Can you work these out from the model? Positions are in its coordinate system, mm. A direction names the side the tool comes from. Give positions to 0.01 mm unless a question says otherwise; leave off trailing zeros. Loops run counter-clockwise (first coordinate to the right, second up) from the corner with the lowest first, then second, coordinate; pieces in that order, holes last. Notation, with made-up numbers: M -38,20.25 L -10,20.25 A35 ccw -10,54.25 Z; hole C 89,-26.5 d9. An arc over 180 degrees is marked long. Answer as a JSON object with one key per item and string values.
Autodesk Inventor part; units mm, degrees
ref_plane "YZ Plane" through (0, 0, 0) normal (1, 0, 0) x (0, 1, 0)
ref_plane "XZ Plane" through (0, 0, 0) normal (0, 1, 0) x (-1, 0, 0)
ref_plane "XY Plane" through (0, 0, 0) normal (0, 0, 1) x (1, 0, 0)
sketch "스케치1" plane through (0, 0, 0) normal (0, 1, 0) x (-1, 0, 0)
  line L0 (60, 75) -> (-60, 75)
  line L1 (-60, 75) -> (-60, -75)
  line L2 (-60, -75) -> (60, -75)
  line L3 (60, -75) -> (60, 75)
  line L4 (60, 75) -> (-60, -75) construction
  line L5 (-60, 75) -> (60, -75) construction
  point P0 (0, 0)
  dimension "d0" = 120
  dimension "d1" = 150
extrude "돌출1" add sketch "스케치1" along normal blind 40
sketch "스케치2" plane through (0, 40, 0) normal (0, 1, 0) x (1, 0, 0)
  line L0 (60, -75) -> (60, 75)
  line L1 (60, 75) -> (-60, 75)
  line L2 (50, 102.1646) -> (-50, 102.1646)
  line L3 (-50, 102.1646) -> (-50, -103.0725)
  line L4 (-50, -103.0725) -> (50, -103.0725)
  line L5 (50, -103.0725) -> (50, 102.1646)
  line L6 (-60, 75) -> (-60, -75)
  point P0 (0, 0)
  point P1 (50, 75)
  point P2 (-50, 75)
  dimension "d6" = 10
  dimension "d7" = 10
extrude "돌출2" cut sketch "스케치2" against normal blind 20 contours L5 L4 L3 L1
sketch "스케치3" plane through (60, 0, 75) normal (1, 0, 0) x (0, 0, -1)
  circle A0 centre (29.6769, 5) radius 14
  circle A1 centre (120, 5) radius 14
  line L0 (150, 0) -> (150, 40)
  line L1 (0, 0) -> (150, 0)
  point P0 (75, 0)
  dimension "d10" = 28
  dimension "d12" = 28
  dimension "d13" = 30
  dimension "d16" = 5
  dimension "d30" = 5
extrude "돌출3" cut sketch "스케치3" against normal blind 19 contours A0 L1 | L1 A0
sketch "스케치4" plane through (60, 0, -75) normal (1, 0, 0) x (0, 0, -1)
  arc A0 (-107.2464, 0) -> (-133.3998, 0) centre (-120.3231, 5) ccw
  line L0 (-134.3231, 36.9687) -> (-106.3231, 36.9687)
  line L1 (-106.3231, 36.9687) -> (-106.3231, -26.9687)
  line L2 (-106.3231, -26.9687) -> (-134.3231, -26.9687)
  line L3 (-134.3231, -26.9687) -> (-134.3231, 36.9687)
  line L4 (-134.3231, 36.9687) -> (-106.3231, -26.9687) construction
  line L5 (-106.3231, 36.9687) -> (-134.3231, -26.9687) construction
  line L6 (-150, 0) -> (-133.3998, 0)
  line L7 (-107.2464, 0) -> (0, 0)
  point P0 (-75, 0)
  point P1 (-134.3231, 0)
  point P2 (-134.3231, 5)
  point P3 (-106.3231, 0)
  point P4 (-106.3231, 5)
  dimension "d17" = 28
extrude "돌출4" cut sketch "스케치4" against normal blind 19 contours A0 L1 L7 | A0 L6 L3
sketch "스케치5" plane through (60, 0, -75) normal (1, 0, 0) x (0, 0, -1)
  line L0 (-127.8231, 12) -> (-112.8231, 12)
  line L1 (-112.8231, 12) -> (-112.8231, 24)
  line L2 (-112.8231, 24) -> (-127.8231, 24)
  line L3 (-127.8231, 24) -> (-127.8231, 12)
  line L4 (-127.8231, 12) -> (-112.8231, 24) construction
  line L5 (-112.8231, 12) -> (-127.8231, 24) construction
  arc A0 (-106.3231, 5) -> (-134.3231, 5) centre (-120.3231, 5) ccw
  point P0 (-75, 0)
  point P1 (-120.3231, 18)
  point P2 (-120.3231, 10)
  dimension "d20" = 15
  dimension "d32" = 19
  dimension "d33" = 0
extrude "돌출5" cut sketch "스케치5" against normal blind 19
sketch "스케치6" plane through (60, 0, -75) normal (1, 0, 0) x (0, 0, -1)
  arc A0 (-106.3231, 5) -> (-134.3231, 5) centre (-120.3231, 5) ccw
  point P0 (-75, 0)
  point P1 (-127.8231, 16.8216)
sketch "스케치7" plane through (60, 0, -75) normal (1, 0, 0) x (0, 0, -1)
  circle A0 centre (-120.3231, 5) radius 17.5 construction
  circle A1 centre (-102.8231, 5) radius 2.1
  circle A2 centre (-137.8231, 5) radius 2.1
  point P0 (-75, 0)
  dimension "d34" = 35
  dimension "d35" = 4.2
  dimension "d36" = 4.2
extrude "돌출6" cut sketch "스케치7" against normal blind 19
mirror "미러1" about plane through (0, 0, 0) normal (1, 0, 0) of "돌출6", "돌출5", "돌출4", "돌출3"
sketch "스케치8" plane through (0, 0, 0) normal (0, -1, 0) x (1, 0, 0)
  line L0 (-41, -88.7468) -> (41, -88.7468)
  line L1 (41, -88.7468) -> (41, 88.7468)
  line L2 (41, 88.7468) -> (-41, 88.7468)
  line L3 (-41, 88.7468) -> (-41, -88.7468)
  line L4 (-41, -88.7468) -> (41, 88.7468) construction
  line L5 (41, -88.7468) -> (-41, 88.7468) construction
  line L6 (41, 31.3231) -> (41, 59.3231)
  point P0 (0, 0)
  dimension "d39" = 0
extrude "돌출7" cut sketch "스케치8" against normal blind 10
sketch "스케치9" plane through (0, 20, 0) normal (0, 1, 0) x (1, 0, 0)
  line L0 (-28.9457, -65) -> (24.4543, -65)
  line L1 (24.4543, -65) -> (24.4543, 3.6)
  line L2 (24.4543, 3.6) -> (-28.9457, 3.6)
  line L3 (-28.9457, 3.6) -> (-28.9457, -65)
  line L4 (50, -75) -> (-50, -75)
  circle A0 centre (-26.3957, -49.7) radius 1.6
  circle A1 centre (21.9043, -51.03) radius 1.6
  circle A2 centre (16.8243, 1.05) radius 1.6
  circle A3 centre (-11.1057, 1.05) radius 1.6
  point P0 (0, 0)
  dimension "d42" = 53.4
  dimension "d43" = 68.6
  dimension "d44" = 10
  dimension "d45" = 3.2
  dimension "d46" = 15.3
  dimension "d47" = 2.55
  dimension "d51" = 3.2
  dimension "d52" = 2.55
  dimension "d56" = 13.97
  dimension "d57" = 3.2
  dimension "d58" = 7.63
  dimension "d59" = 2.55
  dimension "d60" = 3.2
  dimension "d61" = 2.55
  dimension "d62" = 35.56
extrude "돌출8" cut sketch "스케치9" against normal through all contours A0 | A1 | A2 | A3
sketch "스케치10" plane through (0, 20, 0) normal (0, 1, 0) x (1, 0, 0)
  line L0 (50, -75) -> (-50, -75)
  line L1 (2.7, 12.7) -> (45, 12.7)
  line L2 (45, 12.7) -> (45, 55)
  line L3 (45, 55) -> (2.7, 55)
  line L4 (2.7, 55) -> (2.7, 12.7)
  line L5 (-50, -75) -> (-50, 75)
  line L6 (50, 75) -> (50, -75)
  line L7 (39.35, 18.35) -> (8.35, 18.35)
  line L8 (8.35, 18.35) -> (8.35, 49.35)
  line L9 (8.35, 49.35) -> (39.35, 49.35)
  line L10 (39.35, 49.35) -> (39.35, 18.35)
  line L11 (39.35, 18.35) -> (8.35, 49.35) construction
  line L12 (8.35, 18.35) -> (39.35, 49.35) construction
  line L13 (-50, 75) -> (50, 75)
  circle A0 centre (8.35, 49.35) radius 1.6
  circle A1 centre (8.35, 18.35) radius 1.6
  circle A2 centre (39.35, 18.35) radius 1.6
  circle A3 centre (39.35, 49.35) radius 1.6
  point P0 (0, 0)
  point P1 (23.85, 33.85)
  dimension "d68" = 42.3
  dimension "d69" = 42.3
  dimension "d71" = 5
  dimension "d72" = 31
  dimension "d73" = 31
  dimension "d75" = 21.15
  dimension "d76" = 21.15
  dimension "d77" = 20
  dimension "d79" = 3.2
  dimension "d80" = 3.2
  dimension "d81" = 3.2
  dimension "d82" = 3.2
extrude "돌출9" cut sketch "스케치10" against normal through all contours A1 L8 L7 | L7 L8 A1 | A2 L10 L7 | L7 L10 A2 | A0 L9 L8 | L8 L9 A0 | A3 L9 L10 | L10 L9 A3
mirror "미러2" about plane through (0, 0, 0) normal (1, 0, 0) of "돌출9"
properties part number "본체판(구)"
1) Suppose I cut it at C-C, the plane z = 46. Write out the boundary of the cut face in (x, y).
Answer list:
{"outline": "M -60,24 L -50,24 L -50,40 L -60,40 Z; M -41,10 L 41,10 L 41,20 L -41,20 Z; M 50,24 L 60,24 L 60,40 L 50,40 Z"}
2) If we mould it in two halves opening along Z, with no side actions, what happens to faces 4 (the flat face through (51, 0, -21)), 5 (the cylindrical face through (-39, 15.07, -19.91))? For each: +Z half, -Z half, draft (parallel to the pull), parting line (faces both ways), or undercut.
Answer list:
{"face 4": "draft", "face 5": "undercut"}
3) Suppose I cut it at A-A, the plane y = 30.5. Write out the boundary of the cut face in (x, z).
Answer list:
{"outline": "M -60,-75 L -50,-75 L -50,75 L -60,75 Z; M 50,-75 L 60,-75 L 60,75 L 50,75 Z"}
4) Suppose I cut it at D-D, the plane x = -32.5. Write out the boundary of the cut face in (y, z), and give its area (3 significant figures).
Answer list:
{"outline": "M 10,-75 L 20,-75 L 20,75 L 10,75 Z", "area": "1,500 mm^2"}
5) Will these pins go through, and if not, where does the flat tip stop? pin 1 Ø8 at (x, z) = (53, 48.5) entering from -Y; pin 2 Ø6 at (x, z) = (21, 0) entering from -Y; pin 3 Ø4 at (x, z) = (-39.35, -49.35) entering from +Y.
Answer list:
{"pin 1": "y = 24", "pin 2": "y = 10", "pin 3": "y = 20"}
6) For faces 1 (the flat face through (-41, 5, 67)), 2 (the flat face through (-55, 24, 45)), 3 (the cylindrical face through (50.63, 11.66, 33.01)), which set-ups out of +Z, -Z, +X, -X, +Y, -Y let a thin tool reach every point of the face, with its end or its side?
Answer list:
{"face 1": "+Z, -Z, -Y", "face 2": "+X, -X, -Y", "face 3": "+X, -Y"}
7) Please list where these lines run through material, in increasing order: line 1 along X through (y, z) = (13, -1.05); line 2 along Z through (x, y) = (39, 12); line 3 along X through (y, z) = (17, -18). Write a range as from..to.
Answer list:
{"line 1": "-60..-12.71, -9.51..15.22, 18.42..60", "line 2": "-75..-50.91, -47.79..-19.91, -16.79..75", "line 3": "-60..-40.91, -37.79..-9.91, -6.79..6.79, 9.91..37.79, 40.91..60"}
8) Suppose I cut it at B-B, the plane x = 8.35. Write out the boundary of the cut face in (y, z), and give its area (3 significant figures).
Answer list:
{"outline": "M 10,-75 L 20,-75 L 20,-50.95 L 10,-50.95 Z; M 10,-47.75 L 20,-47.75 L 20,-19.95 L 10,-19.95 Z; M 10,-16.75 L 20,-16.75 L 20,75 L 10,75 Z", "area": "1,440 mm^2"}
